Work out the finished part from the listing and answer in its coordinate system (mm). Face numbers are marked on the shaded views. A direction names the side the tool comes from. Round coordinates to 2 decimals unless told otherwise and drop trailing zeros. Loops run counter-clockwise (first coordinate to the right, second up) from the corner with the lowest first, then second, coordinate; pieces in that order, holes last. Notation, with made-up numbers: (65.5, 25) -> (108.5, 25) arc R17 cw to (108.5, 30) -> close; hole circle Ø7 at (85.25, 40). An arc over 180 degrees is marked (long way). Use one line per item in the form item = value.
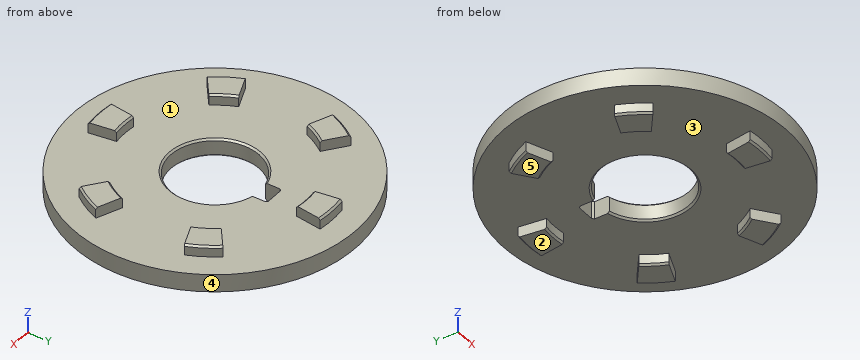
```python
from build123d import *

# Parameters (mm, degrees)
SKETCH1_R                = 80
BOSS_EXTRUDE1_DEPTH      = 5
BOSS_EXTRUDE2_DEPTH      = 6
CHAMFER1_SIZE            = 1
CHAMFER1_OF_MIRROR1_SIZE = 1
CHAMFER2_SIZE            = 1
CHAMFER3_SIZE            = 1


with BuildPart() as part:
    # Sketch1 → Boss-Extrude1 (new body, symmetric)
    with BuildSketch(Plane.XY):
        Circle(SKETCH1_R)
        with BuildLine():
            Line((6, 24.269322199), (6, 33.6))
            Line((6, 33.6), (-6, 33.6))
            Line((-6, 33.6), (-6, 24.269322199))
            ThreePointArc((-6, 24.269322199), (0, -25), (6, 24.269322199))
        make_face(mode=Mode.SUBTRACT)
    extrude(amount=BOSS_EXTRUDE1_DEPTH, both=True)

    # Sketch2 → Boss-Extrude2 (add)
    with BuildSketch(Plane.XY.offset(5)):
        with BuildLine():
            ThreePointArc((-6.97050931, 50.773757985), (0, 51.25), (6.97050931, 50.773757985))
            Line((6.97050931, 50.773757985), (9.010658377, 65.634370079))
            ThreePointArc((9.010658377, 65.634370079), (0, 66.25), (-9.010658377, 65.634370079))
            Line((-9.010658377, 65.634370079), (-6.97050931, 50.773757985))
        make_face()
        with BuildLine():
            ThreePointArc((40.486109606, 31.423517133), (44.383801944, 25.625), (47.456618916, 19.350240853))
            Line((47.456618916, 19.350240853), (61.346361038, 25.01372598))
            ThreePointArc((61.346361038, 25.01372598), (57.374183001, 33.125), (52.335702661, 40.620644098))
            Line((52.335702661, 40.620644098), (40.486109606, 31.423517133))
        make_face()
        with BuildLine():
            ThreePointArc((47.456618916, -19.350240853), (44.383801944, -25.625), (40.486109606, -31.423517133))
            Line((40.486109606, -31.423517133), (52.335702661, -40.620644098))
            ThreePointArc((52.335702661, -40.620644098), (57.374183001, -33.125), (61.346361038, -25.01372598))
            Line((61.346361038, -25.01372598), (47.456618916, -19.350240853))
        make_face()
        with BuildLine():
            ThreePointArc((6.97050931, -50.773757985), (0, -51.25), (-6.97050931, -50.773757985))
            Line((-6.97050931, -50.773757985), (-9.010658377, -65.634370079))
            ThreePointArc((-9.010658377, -65.634370079), (0, -66.25), (9.010658377, -65.634370079))
            Line((9.010658377, -65.634370079), (6.97050931, -50.773757985))
        make_face()
        with BuildLine():
            ThreePointArc((-40.486109606, -31.423517133), (-44.383801944, -25.625), (-47.456618916, -19.350240853))
            Line((-47.456618916, -19.350240853), (-61.346361038, -25.01372598))
            ThreePointArc((-61.346361038, -25.01372598), (-57.374183001, -33.125), (-52.335702661, -40.620644098))
            Line((-52.335702661, -40.620644098), (-40.486109606, -31.423517133))
        make_face()
        with BuildLine():
            ThreePointArc((-47.456618916, 19.350240853), (-44.383801944, 25.625), (-40.486109606, 31.423517133))
            Line((-40.486109606, 31.423517133), (-52.335702661, 40.620644098))
            ThreePointArc((-52.335702661, 40.620644098), (-57.374183001, 33.125), (-61.346361038, 25.01372598))
            Line((-61.346361038, 25.01372598), (-47.456618916, 19.350240853))
        make_face()
    boss_extrude2 = extrude(amount=BOSS_EXTRUDE2_DEPTH)

    # Chamfer1
    chamfer1_edges = [part.edges().sort_by_distance(p)[0] for p in [
        (0, 51.25, 11),
        (0, 66.25, 11),
        (44.383801944, 25.625, 11),
        (57.374183001, 33.125, 11),
        (44.383801944, -25.625, 11),
        (57.374183001, -33.125, 11),
        (0, -51.25, 11),
        (0, -66.25, 11),
        (-44.383801944, -25.625, 11),
        (-57.374183001, -33.125, 11),
        (-44.383801944, 25.625, 11),
        (-57.374183001, 33.125, 11),
    ]]
    chamfer(chamfer1_edges, length=CHAMFER1_SIZE)

    # Mirror1: Boss-Extrude2 across plane
    add(boss_extrude2.mirror(Plane.XY))

    # Chamfer1 of Mirror1
    chamfer1_of_mirror1_edges = [part.edges().sort_by_distance(p)[0] for p in [
        (0, 51.25, -11),
        (0, 66.25, -11),
        (44.383801944, 25.625, -11),
        (57.374183001, 33.125, -11),
        (44.383801944, -25.625, -11),
        (57.374183001, -33.125, -11),
        (0, -51.25, -11),
        (0, -66.25, -11),
        (-44.383801944, -25.625, -11),
        (-57.374183001, -33.125, -11),
        (-44.383801944, 25.625, -11),
        (-57.374183001, 33.125, -11),
    ]]
    chamfer(chamfer1_of_mirror1_edges, length=CHAMFER1_OF_MIRROR1_SIZE)

    # Chamfer2
    chamfer2_edges = [part.edges().sort_by_distance(p)[0] for p in [
        (0, -25, 5),
        (0, -25, -5),
    ]]
    chamfer(chamfer2_edges, length=CHAMFER2_SIZE)

    # Chamfer3
    chamfer3_edges = [part.edges().sort_by_distance(p)[0] for p in [
        (6, 33.6, 0),
        (-6, 33.6, 0),
    ]]
    chamfer(chamfer3_edges, length=CHAMFER3_SIZE)


solid = part.part
```
(1) Given P1, Ø12, axis at x = -52, z = -4.5, coming from the -Y side; P2, Ø4, axis at x = 48, z = 0.5, coming from the +Y side; P3, Ø1, axis at x = -4.5, z = 3.5, coming from the +Y side, each flat-ended and moving along its own axis, determine where each tip first touches the part or whether it passes through.
Completed:
P1 = -65.45
P2 = 65.45
P3 = 79.9
(2) Consider L1, parallel to Y at x = 0, z = 0.75; L2, parallel to Z at x = -29.5, y = -49; L3, parallel to Y at x = 2.5, z = -0.25. Determine where each line is inside the solid, lowest interval first.
Completed:
L1 = -80 to -25, 33.6 to 80
L2 = -5 to 5
L3 = -79.96 to -24.87, 33.6 to 79.96
(3) Find section C-C, the plane z = 1.5. Write down the section's boundary in (x, y), then the cut area to 3 significant figures.
Completed:
outline = circle Ø160 at (0, 0); hole (-6, 24.27) arc R25 ccw (long way) to (6, 24.27) -> (6, 32.6) -> (5, 33.6) -> (-5, 33.6) -> (-6, 32.6) -> close
area = 18,000 mm2
(4) Find section A-A, the plane y = 0. Write down the section's boundary in (x, z).
Completed:
outline = (-80, -5) -> (-26, -5) -> (-25, -4) -> (-25, 4) -> (-26, 5) -> (-80, 5) -> close; (25, -4) -> (26, -5) -> (80, -5) -> (80, 5) -> (26, 5) -> (25, 4) -> close
(5) For the marked faces 1 and 2, determine the directions among +Z, -Z, +X, -X, +Y, -Y from which every point of the face is accessible in a straight line to the end or side of a thin tool.
Completed:
face_1 = +Z
face_2 = -Z, +X, -X, +Y, -Y
(6) For a pull along X with two mould halves and no side action, classify the marked faces 3, 4 and 5 as +X half, -X half, draft (parallel to the pull), parting line (faces both ways), or undercut.
Completed:
face_3 = undercut
face_4 = parting line
face_5 = draft
(7) Find section D-D, the plane y = -43.5. Write down the section's boundary in (x, z).
Completed:
outline = (-67.14, -5) -> (67.14, -5) -> (67.14, 5) -> (-67.14, 5) -> close
